Autodesk Inventor part; units mm, degrees
ref_plane "YZ Plane" through (0, 0, 0) normal (1, 0, 0) x (0, 1, 0)
ref_plane "XZ Plane" through (0, 0, 0) normal (0, 1, 0) x (-1, 0, 0)
ref_plane "XY Plane" through (0, 0, 0) normal (0, 0, 1) x (1, 0, 0)
sketch "Sketch1" plane through (0, 0, 0) normal (0, 1, 0) x (-1, 0, 0)
  line L0 (0, 17.4625) -> (0, 17.4625) construction
  line L1 (0, 17.4625) -> (0, -17.4625) construction
  line L2 (0, -17.4625) -> (0, -17.4625) construction
  line L3 (0, -17.4625) -> (0, 17.4625) construction
  line L4 (0, 17.4625) -> (0, -17.4625) construction
  line L5 (0, 17.4625) -> (0, -17.4625) construction
  circle A0 centre (0, 17.4625) radius 1.7526
  circle A1 centre (0, -17.4625) radius 1.7526
  circle A2 centre (0, 17.4625) radius 1.7526
  circle A3 centre (0, -17.4625) radius 1.7526
  line L6 (-6.35, 28.575) -> (6.35, 28.575)
  line L7 (6.35, 28.575) -> (6.35, -28.575)
  line L8 (6.35, -28.575) -> (-6.35, -28.575)
  line L9 (-6.35, -28.575) -> (-6.35, 28.575)
  line L10 (-6.35, 28.575) -> (6.35, -28.575) construction
  line L11 (6.35, 28.575) -> (-6.35, -28.575) construction
  line L12 (6.35, 28.575) -> (12.7, 28.575)
  line L13 (12.7, 28.575) -> (12.7, -28.575)
  line L14 (12.7, -28.575) -> (6.35, -28.575)
  line L15 (6.35, -28.575) -> (6.35, 28.575)
  line L16 (6.35, 12.7) -> (12.7, 19.05)
  line L17 (6.35, 0) -> (12.7, 0) construction
  line L18 (6.35, -12.7) -> (12.7, -19.05)
  point P0 (0, 0)
  point P1 (12.7, -19.05)
  dimension "d0" = 0
  dimension "d1" = 34.925
  dimension "d2" = 3.5052
  dimension "d5" = 34.925
  dimension "d8" = 0
  dimension "d11" = 12.7
  dimension "d12" = 57.15
  dimension "d40" = 6.35
  dimension "d41" = 9.525
  dimension "d42" = 12.7
extrude "Extrusion1" add sketch "Sketch1" along normal blind 9.525 contours L6 L7 L8 L9 | L12 L13 L16 L7 | L7 L18 L13 L14
sketch "Sketch2" plane through (6.35, 0, 28.575) normal (1, 0, 0) x (0, 0, -1)
  line L0 (28.575, 0) -> (28.575, 9.525) construction
  line L1 (41.275, 9.525) -> (15.875, 9.525)
  circle A0 centre (28.575, 4.7625) radius 3.175
  line L2 (0, 0) -> (57.15, 0)
  point P0 (57.15, 9.525)
  point P1 (0, 9.525)
  point P2 (25.4, 0)
  point P3 (16.2434, 0)
  dimension "d15" = 6.35
  dimension "d16" = 4.7625
extrude "Extrusion2" cut sketch "Sketch2" against normal through all
sketch "Sketch5" plane through (6.35, 0, 28.575) normal (1, 0, 0) x (0, 0, -1)
  line L0 (0, 0) -> (0, 9.525)
  line L1 (0, 4.7625) -> (57.15, 4.7625) construction
  line L2 (57.15, 0) -> (57.15, 9.525)
  line L3 (22.575, 4.7625) -> (34.575, 4.7625) construction
  line L4 (22.575, 3.2625) -> (34.575, 3.2625)
  line L5 (34.575, 6.2625) -> (22.575, 6.2625)
  arc A0 (22.575, 6.2625) -> (22.575, 3.2625) centre (22.575, 4.7625) ccw
  arc A1 (34.575, 3.2625) -> (34.575, 6.2625) centre (34.575, 4.7625) ccw
  point P0 (28.575, 0)
  point P1 (28.575, 4.7625)
  dimension "d29" = 3
  dimension "d30" = 12
extrude "Extrusion5" cut sketch "Sketch5" against normal blind 3
fillet "Fillet3" radius 1.5 6 edges at (3.35, 6.2625, 4.3992) (3.35, 3.2625, 4.3992) (3.35, 4.7625, 7.5) (3.35, 4.7625, -7.5) (3.35, 3.2625, -4.3992) (3.35, 6.2625, -4.3992)
chamfer "Chamfer1" distance 0.5 angle 45 8 edges at (6.35, 3.2625, -4.3992) (6.35, 4.7625, -7.5) (6.35, 6.2625, -4.3992) (6.35, 7.9375, 0) (6.35, 6.2625, 4.3992) (6.35, 4.7625, 7.5) (6.35, 3.2625, 4.3992) (6.35, 1.5875, 0)
fillet "Fillet4" radius 6.35 4 edges at (-6.35, 4.7625, 12.7) (-6.35, 4.7625, -12.7) (-12.7, 4.7625, 19.05) (-12.7, 4.7625, -19.05)
ref_plane "Work Plane1" through (6.35, 0, 0) normal (0, 0, -1) x (-1, 0, 0)
sketch "Sketch6" plane through (6.35, 0, -28.575) normal (0, 0, -1) x (-1, 0, 0)
  line L0 (0, 0) -> (0, 9.525)
  line L1 (0, 4.7625) -> (19.05, 4.7625) construction
  line L2 (19.05, 0) -> (19.05, 9.525)
  line L3 (4.7625, 4.7625) -> (14.2875, 4.7625) construction
  line L4 (4.7625, 2.3813) -> (14.2875, 2.3812)
  line L5 (14.2875, 7.1437) -> (4.7625, 7.1438)
  arc A0 (4.7625, 7.1438) -> (4.7625, 2.3813) centre (4.7625, 4.7625) ccw
  arc A1 (14.2875, 2.3812) -> (14.2875, 7.1437) centre (14.2875, 4.7625) ccw
  circle A2 centre (4.7625, 4.7625) radius 1.65
  circle A3 centre (14.2875, 4.7625) radius 1.65
  point P0 (6.35, 0)
  point P1 (9.525, 4.7625)
  dimension "d44" = 4.7625
  dimension "d45" = 4.7625
  dimension "d46" = 4.7625
  dimension "d47" = 3.3
  dimension "d48" = 3.3
extrude "Extrusion6" add sketch "Sketch6" along normal blind 6.35
mirror "Mirror1" about plane through (6.35, 0, 0) normal (0, 0, -1) of "Extrusion6"
equation "\"d5\" = d1"
equation "\"d45\" = d44"
equation "\"d46\" = d44"
properties part number "Rack - Top" material "Aluminum 6061"
Work out the finished part from the listing and answer in its coordinate system (mm). A direction names the side the tool comes from. Coordinates: 2 decimals unless noted, no trailing zeros. Write each loop counter-clockwise with the first axis right and the second up, starting at its lowest first coordinate (ties: lowest second). Pieces come first, ordered by that corner, then holes.
Q1. Determine the mould class of faces 4 (the face through (-3, 5, -34.925)), 5 (the face through (-7.58, 6.373, -31.706)), 6 (the face through (-12.23, 4.83, -19.28)) for opening direction X: released by +X, released by -X, zero draft, split by the parting line, or undercut.
Q2. Which of the six approach directions +Z, -Z, +X, -X, +Y, -Y give full straight-line access (tool end or side, diameter ignored) to faces 1 (the face through (5.992, 8.08, -0.05)), 2 (the face through (3.97, 4.81, 31.71)), 3 (the face through (-6.35, 2, 2))?
Q3. A cutting plane is placed at C-C, the plane z = 31.5. Give the vertices of the cut face in (x, y).
Q4. Find the intervals of material crossed by line 1 (Z direction, x = 0, y = 5.75) (3 decimals); line 2 (Z direction, x = -1, y = 2) (3 decimals); line 3 (Z direction, x = -2, y = 4.5) (3 decimals), in increasing order.
Q5. Each of these flat-tipped pins is pushed along its axis until it touches: pin 1 Ø3 at (y, z) = (5.5, -6) entering from -X; pin 2 Ø2.5 at (x, y) = (1.5, 5) entering from -Z (3 decimals); pin 3 Ø5.5 at (y, z) = (4.76, 0) entering from -X; pin 4 Ø2 at (x, y) = (1.59, 4.76) entering from +Z (3 decimals). Where does it stop, or does it pass through?
Findings below:
1. face 4: zero draft
1. face 5: undercut
1. face 6: released by -X
2. face 1: +X
2. face 2: +Z, +X
2. face 3: -X, +Y, -Y
3. outline: (-7.94, 2.38) - (1.59, 2.38) arc R2.38 ccw to (1.59, 7.14) - (-7.94, 7.14) arc R2.38 ccw to start; hole circle Ø3.3 at (-7.94, 4.76); hole circle Ø3.3 at (1.59, 4.76)
4. line 1: z = -34.925 to -19.215, -15.71 to -3.018, 3.018 to 15.71, 19.215 to 34.925
4. line 2: z = -28.575 to -18.902, -16.023 to -1.565, 1.565 to 16.023, 18.902 to 28.575
4. line 3: z = -34.925 to -3.164, 3.164 to 34.925
5. pin 1: stops at x = -6.35
5. pin 2: stops at z = -28.575
5. pin 3: passes through
5. pin 4: stops at z = 28.575
